Check sheet for the modelled part. Datum: model origin and axes. Units: mm. A direction names the side the tool comes from. Give positions to 0.01 mm unless a question says otherwise; leave off trailing zeros. Write each loop counter-clockwise with the first axis right and the second up, starting at its lowest first coordinate (ties: lowest second). Pieces come first, ordered by that corner, then holes. Notation, with made-up numbers: M -36,11.5 L 23,11.5 A29 ccw 23,50.5 Z; hole C 29.5,0.5 d4. An arc over 180 degrees is marked long. Use CSV: the item, a comma, the result in double quotes. Start each with the question number.
1. Cross-section at D-D, the plane z = 0. Enter the section's corners in (x, y).
2. Cross-section at B-B, the plane z = -6. Enter the section's corners in (x, y), and give its area (3 significant figures).
3. Cross-section at A-A, the plane y = 0. Enter the section's corners in (x, z).
4. Cross-section at C-C, the plane x = 8. Enter the section's corners in (y, z).
5. Scan lines: line 1 (Y direction, x = 8.5, z = 0); line 2 (X direction, y = -21, z = -13). Record each from-to range of solid material in increasing order.
6. Access from +Z, -Z, +X, -X, +Y, -Y to the whole of each face (thin tool, end or side, straight path). Record for faces 1 (the face through (-21, -21, -15.149)), 2 (the face through (0, -22, 0)), 3 (the face through (-21, -22, 15.149)), 4 (the face through (-42, -23, 0)).
7. Depth check by flat-ended pin: P1, Ø6, axis at x = -4.5, y = -7, coming from the +Z side; P2, Ø6, axis at x = -33.5, z = -13, coming from the +Y side; P3, Ø1.5, axis at y = -23.5, z = -0.5, coming from the +X side; P4, Ø1.7, axis at x = -24.5, y = -21.5, coming from the -Z side. Enter the tip coordinate at first touch or a pass-through.
8. Mould release check, pull along Y, two halves, no side actions. Record for faces 5 (the face through (21.1, 24.3, 8.2)), 6 (the face through (-21, -20.45, 0)), 7 (the face through (10.7, 21.46, -13.68)): +Y half, -Y half, draft (parallel to the pull), parting line (faces both ways), or undercut.
from build123d import *

# Parameters (mm, degrees)
SKETCH1_R           = 27.15
BOSS_EXTRUDE1_DEPTH = 21.1
SKETCH2_R           = 25.45
CUT_EXTRUDE1_DEPTH  = 21.1
BOSS_EXTRUDE3_DEPTH = 42


with BuildPart() as part:
    # Sketch1 → Boss-Extrude1 (new body)
    with BuildSketch(Plane(origin=(0, 0, 0), x_dir=(0, 0, -1), z_dir=(1, 0, 0))):
        Circle(SKETCH1_R)
    extrude(amount=BOSS_EXTRUDE1_DEPTH)

    # Sketch2 → Cut-Extrude1 (cut)
    with BuildSketch(Plane(origin=(21.1, 0, 0), x_dir=(0, 0, -1), z_dir=(1, 0, 0))):
        Circle(SKETCH2_R)
    extrude(amount=-CUT_EXTRUDE1_DEPTH, mode=Mode.SUBTRACT)

    # Sketch3 → Boss-Extrude3 (add)
    with BuildSketch(Plane.ZY):
        with BuildLine():
            Line((0, -20.45), (-15.149257408, -20.45))
            Line((-15.149257408, -20.45), (-15.149257408, -22.530479356))
            ThreePointArc((-15.149257408, -22.530479356), (0, -27.15), (15.149257408, -22.530479356))
            Line((15.149257408, -22.530479356), (15.149257408, -20.45))
            Line((15.149257408, -20.45), (0, -20.45))
        make_face()
    extrude(amount=BOSS_EXTRUDE3_DEPTH)


solid = part.part
Worked answers:
1,outline,"M -42,-27.15 L 21.1,-27.15 L 21.1,-25.45 L 0,-25.45 L 0,-20.45 L -42,-20.45 Z; M 0,25.45 L 21.1,25.45 L 21.1,27.15 L 0,27.15 Z"
2,outline,"M -42,-26.48 L 21.1,-26.48 L 21.1,-24.73 L 0,-24.73 L 0,-20.45 L -42,-20.45 Z; M 0,24.73 L 21.1,24.73 L 21.1,26.48 L 0,26.48 Z"
2,area,"327 mm^2"
3,outline,"M 0,-27.15 L 21.1,-27.15 L 21.1,-25.45 L 0,-25.45 Z; M 0,25.45 L 21.1,25.45 L 21.1,27.15 L 0,27.15 Z"
4,outline,"C 0,0 d54.3; hole C 0,0 d50.9"
5,line 1,"y = -27.15 to -25.45, 25.45 to 27.15"
5,line 2,"x = -42 to 0"
6,face 1,"-Z, -X, +Y, -Y"
6,face 2,"+X"
6,face 3,"+Z, -X, +Y, -Y"
6,face 4,"+Z, -Z, -X, +Y, -Y"
7,P1,"passes through"
7,P2,"stops at y = -20.45"
7,P3,"stops at x = 0"
7,P4,"stops at z = -15.15"
8,face 5,"draft"
8,face 6,"+Y half"
8,face 7,"undercut"
